from build123d import *

# Parameters (mm, degrees)
F1_DEPTH = 6.35
F3_D     = 5.08
F4_W     = 3.175
F4_H     = 6.35
F5_DEPTH = 25.4


with BuildPart() as f1:
    # F0 (on Top) → F1 (new body)
    with BuildSketch(Plane.XY):
        Polygon((52.07, 29.21), (52.07, 82.55), (-52.07, 82.55), (-52.07, 29.21), (-25.4, -41.91), (0, -41.91), (25.4, -41.91), align=None)
    extrude(amount=F1_DEPTH)

    # F3 (through all)
    with Locations(Plane.XY.offset(6.35)):
        with Locations((-15.24, -26.67), (15.24, -26.67), (0, 0), (-45.72, 24.13), (-25.4, -24.13), (25.4, -24.13), (45.72, 24.13), (25.4, 76.2), (-25.4, 76.2)):
            Hole(F3_D / 2)

    # F4 (on face) → F5 (cut)
    with BuildSketch(Plane.XY.offset(6.35)):
        with Locations((-47.3075, 60.325)):
            Rectangle(F4_W, F4_H)
        with Locations((47.3075, 60.325)):
            Rectangle(F4_W, F4_H)
        with Locations((-47.3075, 47.625)):
            Rectangle(F4_W, F4_H)
        with Locations((47.3075, 47.625)):
            Rectangle(F4_W, F4_H)
    extrude(amount=-F5_DEPTH, mode=Mode.SUBTRACT)


solid = f1.part
Build history of the part. All positions in model axes, mm. A direction names the side the tool comes from. Coordinates: 2 decimals unless noted, no trailing zeros. Write each loop counter-clockwise with the first axis right and the second up, starting at its lowest first coordinate (ties: lowest second). Pieces come first, ordered by that corner, then holes. Notation, with made-up numbers: (-19, -20) -> (16, -20) arc R22 cw to (16, 0) -> close; hole circle Ø3 at (38.5, 52). An arc over 180 degrees is marked (long way). Use CSV: the item, a comma, the result in double quotes. Start each with the question number.
Q1. 3-axis set-ups, long thin cutter, end or side, ignore diameter. For faces 1 (the flat face through (0, -41.91, 3)), 2 (the flat face through (47, 57.15, 3)): which of +Z, -Z, +X, -X, +Y, -Y reach the whole face in a straight line?
Q2. Cut at C-C, the plane z = 4.5. State how many separate pieces and enclosed holes the cut face has, then the cut area to 3 significant figures.
Q3. Drill centre lines: probe 1 along Y at (x, z) = (-25, 3); probe 2 along X at (y, z) = (46, 3.75) (3 decimals); probe 3 along Y at (x, z) = (15, 3.25). Where is each one in solid material? Low to high.
Q4. Pull direction Y, two halves, no side cores. Call faces 3 (the flat face through (-45.72, 48, 3)), 4 (the flat face through (-38.922, -5.852, 3.131)), 5 (the flat face through (1, 82.55, 3)): released by +Y, released by -Y, zero draft, split by the parting line, or undercut.
Q5. Cut at A-A, the plane x = -15.24. List the corners of the cut face in (y, z).
Q6. Cut at D-D, the plane y = 0. List the corners of the cut face in (x, z).
Q7. Flat gauge pin, fed straight in: pin 1 Ø6.5 at (x, y) = (-25.4, -24.13) entering from +Z. Where does the tip first touch, or does it go through?
Q8. Cut at B-B, the plane y = 48.5. List the corners of the cut face in (x, z) (3 decimals), then the cut area to 3 significant figures.
Checked values:
1,face 1,"+Z, -Z, +X, -X, -Y"
1,face 2,"+Z, -Z"
2,separate pieces,"1"
2,enclosed holes,"13"
2,area,"10,800 mm²"
3,probe 1,"y = -41.91 to -26.64, -21.62 to 73.69, 78.71 to 82.55"
3,probe 2,"x = -52.07 to -48.895, -45.72 to 45.72, 48.895 to 52.07"
3,probe 3,"y = -41.91 to -29.2, -24.14 to 82.55"
4,face 3,"undercut"
4,face 4,"released by -Y"
4,face 5,"released by +Y"
5,outline,"(-41.91, 0) -> (-29.21, 0) -> (-29.21, 6.35) -> (-41.91, 6.35) -> close; (-24.13, 0) -> (82.55, 0) -> (82.55, 6.35) -> (-24.13, 6.35) -> close"
6,outline,"(-41.12, 0) -> (-2.54, 0) -> (-2.54, 6.35) -> (-41.12, 6.35) -> close; (2.54, 0) -> (41.12, 0) -> (41.12, 6.35) -> (2.54, 6.35) -> close"
7,pin 1,"stops at z = 6.35"
8,outline,"(-52.07, 0) -> (-48.895, 0) -> (-48.895, 6.35) -> (-52.07, 6.35) -> close; (-45.72, 0) -> (45.72, 0) -> (45.72, 6.35) -> (-45.72, 6.35) -> close; (48.895, 0) -> (52.07, 0) -> (52.07, 6.35) -> (48.895, 6.35) -> close"
8,area,"621 mm²"
